Read the model definition and answer for the solid it produces. Units are mm, in the model's axes. A direction names the side the tool comes from. Coordinates: 2 decimals unless noted, no trailing zeros. Loops run counter-clockwise (first coordinate to the right, second up) from the corner with the lowest first, then second, coordinate; pieces in that order, holes last.
from build123d import *

# Parameters (mm, degrees)
BOSS_EXTRUDE1_DEPTH = 90
BOSS_EXTRUDE2_DEPTH = 3
SKETCH3_R           = 13.5
BOSS_EXTRUDE3_DEPTH = 90
BOSS_EXTRUDE4_START = -3
BOSS_EXTRUDE4_DEPTH = 3
SKETCH5_R           = 11
CUT_EXTRUDE1_DEPTH  = 200
SCALE1_SCALE        = 1.5
SKETCH6_R           = 25
CUT_EXTRUDE2_DEPTH  = 65
SCALE2_SCALE        = 0.6


# Read off the part's stored shape, not the designer's step: Shell4
with BuildPart() as part:
    # Sketch1 → Boss-Extrude1 (new body)
    with BuildSketch(Plane(origin=(0, 0, 0), x_dir=(1, 0, 0), z_dir=(0, 1, 0))):
        with BuildLine():
            ThreePointArc((-4, 22.141589825), (-22.5, 0), (-4, -22.141589825))
            Line((-4, -22.141589825), (-4, 22.141589825))
        make_face()
        with BuildLine():
            Line((-4, 22.141589825), (-4, -22.141589825))
            ThreePointArc((-4, -22.141589825), (0, -22.5), (4, -22.141589825))
            Line((4, -22.141589825), (4, 22.141589825))
            ThreePointArc((4, 22.141589825), (0, 22.5), (-4, 22.141589825))
        make_face()
        with BuildLine():
            Line((4, 22.141589825), (4, -22.141589825))
            ThreePointArc((4, -22.141589825), (17.26629665, -14.426538046), (22.5, 0))
            ThreePointArc((22.5, 0), (17.26629665, 14.426538046), (4, 22.141589825))
        make_face()
    extrude(amount=BOSS_EXTRUDE1_DEPTH)

    # Sketch1<3> → Boss-Extrude2 (add)
    with BuildSketch(Plane(origin=(0, 0, 0), x_dir=(1, 0, 0), z_dir=(0, 1, 0))):
        with BuildLine():
            Line((-4, 25.5), (-4, 22.141589825))
            ThreePointArc((-4, 22.141589825), (0, 22.5), (4, 22.141589825))
            Line((4, 22.141589825), (4, 25.5))
            Line((4, 25.5), (-4, 25.5))
        make_face()
        with BuildLine():
            Line((-4, -22.141589825), (-4, -25.5))
            Line((-4, -25.5), (4, -25.5))
            Line((4, -25.5), (4, -22.141589825))
            ThreePointArc((4, -22.141589825), (0, -22.5), (-4, -22.141589825))
        make_face()
    extrude(amount=BOSS_EXTRUDE2_DEPTH)

    # Sketch3 → Boss-Extrude3 (add)
    with BuildSketch(Plane(origin=(0, 90, 0), x_dir=(1, 0, 0), z_dir=(0, 1, 0))):
        with Locations(Location((0, 0, 0), (0, 0, 90))):
            Circle(SKETCH3_R)
    extrude(amount=BOSS_EXTRUDE3_DEPTH)

    # Sketch4 → Boss-Extrude4 (add)
    with BuildSketch(Plane(origin=(0, 180, 0), x_dir=(1, 0, 0), z_dir=(0, 1, 0)).offset(BOSS_EXTRUDE4_START)):
        with BuildLine():
            Line((-8.690152284, 12.277265708), (-13.755690181, 6.085309166))
            Line((-13.755690181, 6.085309166), (-12.345874566, 5.461628073))
            ThreePointArc((-12.345874566, 5.461628073), (-10.448926665, 8.5480952), (-7.799501781, 11.018973272))
            Line((-7.799501781, 11.018973272), (-8.690152284, 12.277265708))
        make_face()
        with BuildLine():
            ThreePointArc((-7.799501781, 11.018973272), (-7.62418516, 11.140996394), (-7.446959855, 11.260230411))
            Line((-7.446959855, 11.260230411), (-8.690152284, 12.277265708))
            Line((-8.690152284, 12.277265708), (-7.799501781, 11.018973272))
        make_face()
        with BuildLine():
            ThreePointArc((12.345874566, -5.461628073), (12.430742152, -5.265610084), (12.512497752, -5.068273869))
            Line((12.512497752, -5.068273869), (-7.446959855, 11.260230411))
            ThreePointArc((-7.446959855, 11.260230411), (-7.62418516, 11.140996394), (-7.799501781, 11.018973272))
            Line((-7.799501781, 11.018973272), (0, 0))
            Line((0, 0), (12.345874566, -5.461628073))
        make_face()
        with BuildLine():
            Line((0, 0), (7.799501781, -11.018973272))
            ThreePointArc((7.799501781, -11.018973272), (10.448926665, -8.5480952), (12.345874566, -5.461628073))
            Line((12.345874566, -5.461628073), (0, 0))
        make_face()
        with BuildLine():
            Line((-12.345874566, 5.461628073), (0, 0))
            Line((0, 0), (-7.799501781, 11.018973272))
            ThreePointArc((-7.799501781, 11.018973272), (-10.448926665, 8.5480952), (-12.345874566, 5.461628073))
        make_face()
        with BuildLine():
            Line((-12.512497752, 5.068273869), (7.446959855, -11.260230411))
            ThreePointArc((7.446959855, -11.260230411), (7.62418516, -11.140996394), (7.799501781, -11.018973272))
            Line((7.799501781, -11.018973272), (0, 0))
            Line((0, 0), (-12.345874566, 5.461628073))
            ThreePointArc((-12.345874566, 5.461628073), (-12.430742152, 5.265610084), (-12.512497752, 5.068273869))
        make_face()
        with BuildLine():
            Line((-13.755690181, 6.085309166), (-12.512497752, 5.068273869))
            ThreePointArc((-12.512497752, 5.068273869), (-12.430742152, 5.265610084), (-12.345874566, 5.461628073))
            Line((-12.345874566, 5.461628073), (-13.755690181, 6.085309166))
        make_face()
        with BuildLine():
            Line((12.345874566, -5.461628073), (13.755690181, -6.085309166))
            Line((13.755690181, -6.085309166), (12.512497752, -5.068273869))
            ThreePointArc((12.512497752, -5.068273869), (12.430742152, -5.265610084), (12.345874566, -5.461628073))
        make_face()
        with BuildLine():
            Line((7.799501781, -11.018973272), (8.690152284, -12.277265708))
            Line((8.690152284, -12.277265708), (13.755690181, -6.085309166))
            Line((13.755690181, -6.085309166), (12.345874566, -5.461628073))
            ThreePointArc((12.345874566, -5.461628073), (10.448926665, -8.5480952), (7.799501781, -11.018973272))
        make_face()
        with BuildLine():
            Line((7.446959855, -11.260230411), (8.690152284, -12.277265708))
            Line((8.690152284, -12.277265708), (7.799501781, -11.018973272))
            ThreePointArc((7.799501781, -11.018973272), (7.62418516, -11.140996394), (7.446959855, -11.260230411))
        make_face()
    extrude(amount=BOSS_EXTRUDE4_DEPTH)

    # Sketch2 one side → Revolve1 (revolve)
    with BuildSketch(Plane(origin=(0, 90, 0), x_dir=(1, 0, 0), z_dir=(0, 1, 0))):
        with BuildLine():
            Line((-22.5, 0), (22.5, 0))
            ThreePointArc((22.5, 0), (0, 22.5), (-22.5, 0))
        make_face()
        with BuildLine():
            Line((-75, 0), (75, 0))
            ThreePointArc((75, 0), (0, 75), (-75, 0))
        make_face()
        with BuildLine():
            ThreePointArc((-22.5, 0), (0, -22.5), (22.5, 0))
            Line((22.5, 0), (-22.5, 0))
        make_face()
    revolve(axis=Axis((-75, 90, 0), (1, 0, 0)))

    # Shell4 outline → Shell4 (revolve, cut)
    with BuildSketch(Plane.XY):
        with BuildLine():
            Line((6.499999977, 157.688625339), (6.5, 173))
            Line((6.5, 173), (0, 173))
            Line((0, 173), (0, 7))
            Line((0, 7), (15.5, 7))
            Line((15.5, 7), (15.499999978, 23.790106474))
            ThreePointArc((15.499999978, 23.790106474), (67.846911043, 94.560335727), (6.499999977, 157.688625339))
        make_face()
    revolve(axis=Axis((0, 0, 0), (0, 1, 0)), mode=Mode.SUBTRACT)

    # Sketch5 → Cut-Extrude1 (cut)
    with BuildSketch(Plane(origin=(0, 180, 0), x_dir=(1, 0, 0), z_dir=(0, 1, 0))):
        with Locations(Location((0, 0, 0), (0, 0, 270))):
            Circle(SKETCH5_R)
    extrude(amount=-CUT_EXTRUDE1_DEPTH, mode=Mode.SUBTRACT)


with BuildPart() as part_1:
    # Scale1: scaled about (-7.769e-06, 87.871063755, -1.7236e-05)
    add(part.part.scale(SCALE1_SCALE).moved(Location((3.884e-06, -43.935531877, 8.618e-06))))

    # Sketch6 → Cut-Extrude2 (cut)
    with BuildSketch(Plane.XZ.offset(43.93576905)):
        with Locations(Location((0, 0, 0), (0, 0, 270))):
            Circle(SKETCH6_R)
    extrude(amount=-CUT_EXTRUDE2_DEPTH, mode=Mode.SUBTRACT)


with BuildPart() as part_2:
    # Scale2: scaled about (-8.009e-06, 89.299768171, -1.5386e-05)
    add(part_1.part.scale(SCALE2_SCALE).moved(Location((-3.204e-06, 35.719907268, -6.154e-06))))


solid = part_2.part
Q1. Determine the mould class of faces 4 (the face through (-0.1, 9.359, -15.4)), 5 (the face through (10.07, 169.99, 8.3)), 6 (the face through (-14.643, 20.04, 3.252)) for opening direction X: +X half, -X half, draft (parallel to the pull), parting line (faces both ways), or undercut.
Findings below:
face 4: draft
face 5: +X half
face 6: undercut
Q2. Which of the six approach directions +Z, -Z, +X, -X, +Y, -Y give full straight-line access (tool end or side, diameter ignored) to faces 1 (the face through (4.654, 163.955, -11.224)), 2 (the face through (10, 168.659, 8)), 3 (the face through (-10.07, 169.99, -8.3))?
Findings below:
face 1: none
face 2: +Z, +X
face 3: -Z, -X, +Y
Q3. Flat-ended cylindrical pins translate along their axes: pin 1 Ø1.3 at (x, y) = (-0.5, 10) entering from -Z; pin 2 Ø12 at (y, z) = (123.5, 17) entering from +X; pin 3 Ø3 at (y, z) = (124, -16) entering from +X; pin 4 Ø18 at (x, z) = (0, 0) entering from -Y. Find the tip coordinate at first contact, or state that the pin passes through.
Findings below:
pin 1: stops at z = -22.95
pin 2: stops at x = 59.83
pin 3: stops at x = 57.25
pin 4: passes through
Q4. A cutting plane is placed at A-A (y = 144). Give the vertices of the cut face in (x, z) (1 decimal), then the cut area to 3 significant figures.
Findings below:
outline: circle Ø81.9 at (0, 0); hole circle Ø58.9 at (0, 0)
area: 2,550 mm2
Q5. A cutting plane is placed at B-B (z = -51). Give the vertices of the cut face in (x, y).
Findings below:
outline: circle Ø88.44 at (0, 90.36); hole circle Ø67.66 at (0, 90.36)
Q6. Straight lines are drawn through the part: probe 1 along X at (y, z) = (162.25, 0); probe 2 along Y at (x, z) = (-24.5, -10.5). For each, find the intervals that lie inside material, in ascending order.
Findings below:
probe 1: x = -12.15 to -9.9, 9.9 to 12.15
probe 2: y = 28.34 to 35.27, 145.45 to 152.37
